Verification items for the finished model (mm, model axes). Give positions to 0.01 mm unless a question says otherwise; leave off trailing zeros. Order: outer loops, then holes, each group sorted by start corner. A loop starts at its lowest first (then second) coordinate and runs counter-clockwise, first axis right, second up. Notation, with made-up numbers: (14, 54.5) - (34, 54.5) arc R5 cw to (34, 60.5) - close; hole circle Ø1 at (-17, 22). An arc over 180 degrees is marked (long way). Answer as a JSON object with one key per item and string values.
```python
from build123d import *

# Parameters (mm, degrees)
SKETCH1_W          = 44.45
SKETCH1_H          = 346.075
BASE_FLANGE1_DEPTH = 3.0226
CUT_EXTRUDE1_REACH = 176.485
SKETCH6_R          = 5.159375
SKETCH6_W          = 19.05
SKETCH6_H          = 52.3875
FILLET2_R          = 50.8
FILLET3_R          = 3.175


# Sheet-metal steps are written as plain solids
with BuildPart() as part:
    # Sketch1 → Base-Flange1 (new body)
    with BuildSketch(Plane(origin=(0, 0, 0), x_dir=(1, 0, 0), z_dir=(0, 1, 0))):
        Rectangle(SKETCH1_W, SKETCH1_H)
    extrude(amount=-BASE_FLANGE1_DEPTH)

    # Sketch6 → Cut-Extrude1 (cut, up to next)
    with BuildSketch(Plane(origin=(0, 0, 0), x_dir=(1, 0, 0), z_dir=(0, 1, 0)), mode=Mode.PRIVATE) as cut_extrude1_sk1:
        with Locations(Location((-7.540625, -131.7625, 0), (0, 0, 270))):
            Circle(SKETCH6_R)
    cut_extrude1_tool1 = extrude(cut_extrude1_sk1.sketch, amount=-CUT_EXTRUDE1_REACH, mode=Mode.PRIVATE) & part.part
    # Sketch6 → Cut-Extrude1 (cut, up to next)
    with BuildSketch(Plane(origin=(0, 0, 0), x_dir=(1, 0, 0), z_dir=(0, 1, 0)), mode=Mode.PRIVATE) as cut_extrude1_sk2:
        with Locations(Location((-7.540625, 88.9, 0), (0, 0, 270))):
            Circle(SKETCH6_R)
    cut_extrude1_tool2 = extrude(cut_extrude1_sk2.sketch, amount=-CUT_EXTRUDE1_REACH, mode=Mode.PRIVATE) & part.part
    # Sketch6 → Cut-Extrude1 (cut, up to next)
    with BuildSketch(Plane(origin=(0, 0, 0), x_dir=(1, 0, 0), z_dir=(0, 1, 0)), mode=Mode.PRIVATE) as cut_extrude1_sk3:
        with Locations((12.7, 146.84375)):
            Rectangle(SKETCH6_W, SKETCH6_H)
    cut_extrude1_tool3 = extrude(cut_extrude1_sk3.sketch, amount=-CUT_EXTRUDE1_REACH, mode=Mode.PRIVATE) & part.part
    add(cut_extrude1_tool1.solids().sort_by_distance((-7.540625, 0, 131.7625))[0], mode=Mode.SUBTRACT)
    add(cut_extrude1_tool2.solids().sort_by_distance((-7.540625, 0, -88.9))[0], mode=Mode.SUBTRACT)
    add(cut_extrude1_tool3.solids().sort_by_distance((12.7, 0, -146.84375))[0], mode=Mode.SUBTRACT)

    # Fillet2
    # the kernel refuses this fillet: 50.8 mm, written as the material it adds along each edge
    with BuildSketch(Plane(origin=(3.175, 0, -120.65), x_dir=(1, 0, 0), z_dir=(0, -1, 0))) as fillet2_piece_1:
        with BuildLine():
            CenterArc((50.8, -39.65573729), FILLET2_R, 128.682187453, 51.317812547)
            Line((0, -39.65573729), (-1.016, -39.65573729))
            Line((-1.016, -39.65573729), (-1.016, 0))
            Line((-1.016, 0), (0, 1.016))
            ThreePointArc((0, 1.016), (9.525, 1.016), (18.415, 0.793114746))
            Line((18.415, 0.793114746), (19.05, 0))
        make_face()
    extrude(amount=3.0226)

    # Fillet3
    fillet3_edges = [part.edges().sort_by_distance(p)[0] for p in [
        (22.225, -1.5113, -120.65),
        (3.175, -1.5113, -173.0375),
        (-22.225, -1.5113, -173.0375),
        (22.225, -1.5113, 173.0375),
        (-22.225, -1.5113, 173.0375),
    ]]
    fillet(fillet3_edges, radius=FILLET3_R)


solid = part.part
```
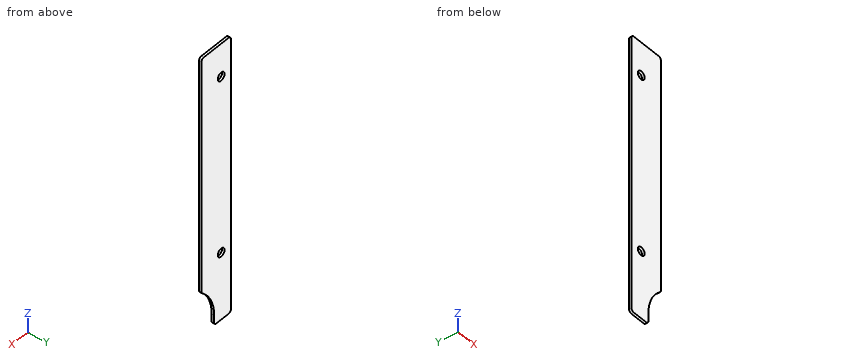
(1) Section check B-B (y = -0.9). Count the separate pieces of the cut face and the enclosed holes in it, then the cut area to 3 significant figures.
Computed values:
{"separate pieces": "1", "enclosed holes": "2", "area": "14,400 mm²"}
(2) Section check A-A (z = -88.9). Record the cut outline in (x, y) (3 decimals), then the cut area to 3 significant figures.
Computed values:
{"outline": "(-22.225, -3.023) - (-12.7, -3.023) - (-12.7, 0) - (-22.225, 0) - close; (-2.381, -3.023) - (22.225, -3.023) - (22.225, 0) - (-2.381, 0) - close", "area": "103 mm²"}
(3) Material ranges on line 1 along Z through (x, y) = (-7.5, -2.1); line 2 along X through (y, z) = (-1.4, -88.9) (3 decimals); line 3 along Z through (x, y) = (-10.5, -2.65), recorded low to high. Write a range as [from, to].
Computed values:
{"line 1": "z = [-173.04, -94.06], [-83.74, 126.6], [136.92, 173.04]", "line 2": "x = [-22.225, -12.7], [-2.381, 22.225]", "line 3": "z = [-173.04, -93.13], [-84.67, 127.54], [135.99, 173.04]"}
